The drawing under review shows one solid part. Ordinate dimensions are in mm from its lowest x, y, z. A direction names the side the tool comes from. Coordinates: 2 decimals unless noted, no trailing zeros. Loops run counter-clockwise (first coordinate to the right, second up) from the corner with the lowest first, then second, coordinate; pieces in that order, holes last. Notation, with made-up numbers: (63, 79.5) - (116, 79.5) arc R12 ccw to (116, 94.5) - close; hole circle Ø4 at (85.25, -19). An arc over 180 degrees is marked (long way). Use one line per item in the form item = value. Start each with the question number.
1. Add section A-A on y = 62.5. Give the boundary of the cut face in (x, z) (3 decimals), and give its area (3 significant figures).
2. Draft analysis for pull direction X (two halves, no side actions). For the marked faces 3, 4 and 5, state which applies: +X half, -X half, draft (parallel to the pull), parting line (faces both ways), or undercut.
3. Add section C-C on x = 27. Give the boundary of the cut face in (y, z) (3 decimals).
4. Machinability: for the marked faces 1 and 2, which of the approach directions +Z, -Z, +X, -X, +Y, -Y give a long, thin tool a straight path to every point of the face, cutting with its end or side? Answer none if there is none.
5. Add section B-B on z = 5.25. Give the boundary of the cut face in (x, y) (3 decimals), and give its area (3 significant figures).
6. To check wall thickness, follow probe 1 along X at (y, z) = (35, 5.5) (3 decimals); probe 2 along Y at (x, z) = (23.5, 6) (3 decimals); probe 3 along X at (y, z) = (74, 3.5) (3 decimals). State the ranges of each line that lie inside material, in increasing order.
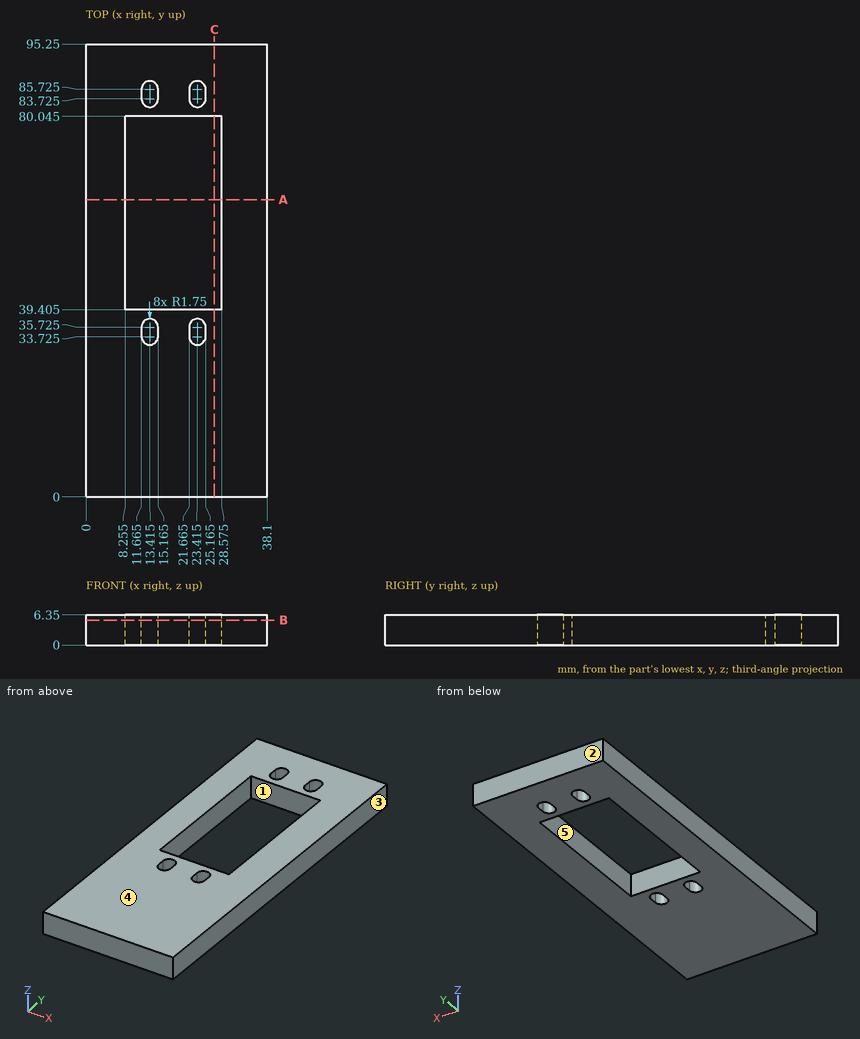
Conclusion:
q1.outline = (0, 0) - (8.255, 0) - (8.255, 6.35) - (0, 6.35) - close; (28.575, 0) - (38.1, 0) - (38.1, 6.35) - (28.575, 6.35) - close
q1.area = 113 mm^2
q2.face_3 = +X half
q2.face_4 = draft
q2.face_5 = undercut
q3.outline = (0, 0) - (39.405, 0) - (39.405, 6.35) - (0, 6.35) - close; (80.045, 0) - (95.25, 0) - (95.25, 6.35) - (80.045, 6.35) - close
q4.face_1 = +Z, -Z
q4.face_2 = +Z, -Z, +X, -X, +Y
q5.outline = (0, 0) - (38.1, 0) - (38.1, 95.25) - (0, 95.25) - close; hole (8.255, 39.405) - (28.575, 39.405) - (28.575, 80.045) - (8.255, 80.045) - close; hole (11.665, 33.725) arc R1.75 ccw to (15.165, 33.725) - (15.165, 35.725) arc R1.75 ccw to (11.665, 35.725) - close; hole (11.665, 83.725) arc R1.75 ccw to (15.165, 83.725) - (15.165, 85.725) arc R1.75 ccw to (11.665, 85.725) - close; hole (21.665, 33.725) arc R1.75 ccw to (25.165, 33.725) - (25.165, 35.725) arc R1.75 ccw to (21.665, 35.725) - close; hole (21.665, 83.725) arc R1.75 ccw to (25.165, 83.725) - (25.165, 85.725) arc R1.75 ccw to (21.665, 85.725) - close
q5.area = 2,740 mm^2
q6.probe_1 = 0 to 11.665, 15.165 to 21.665, 25.165 to 38.1
q6.probe_2 = 0 to 31.977, 37.473 to 39.405, 80.045 to 81.977, 87.473 to 95.25
q6.probe_3 = 0 to 8.255, 28.575 to 38.1
